For this review, use the dimensioned drawing (mm, ordinates from the lowest corner) and the shaded views. Coordinates: 2 decimals unless noted, no trailing zeros. Write each loop counter-clockwise with the first axis right and the second up, starting at its lowest first coordinate (ties: lowest second). Pieces come first, ordered by that corner, then holes. Notation, with made-up numbers: (-22.5, -39) - (23.5, -39) arc R15 ccw to (23.5, -28) - close; hole circle Ø1 at (50, 43). An arc over 180 degrees is marked (long way). One line per item, written item: value.
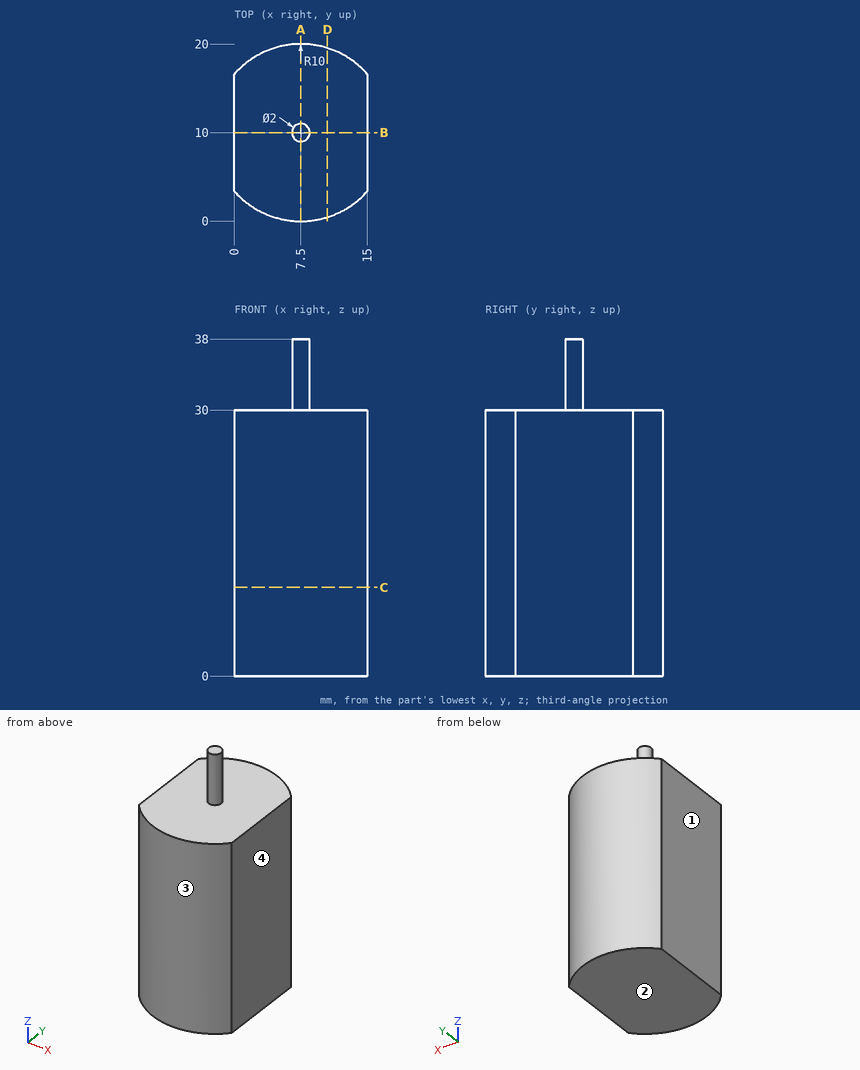
1. Insertion check: pin 1 Ø5 at (x, y) = (13.5, 13) entering from +Z; pin 2 Ø2 at (x, z) = (9, 30.5) entering from +Y. Each pin has a flat end and moves straight along its axis. Give the tip position at first contact, or say it passes through.
Answer block:
pin 1: stops at z = 30
pin 2: stops at y = 19.98
2. Consider section C-C, the plane z = 10. Write out the cut boundary in (x, y), then the cut area to 3 significant figures.
Answer block:
outline: (0, 3.39) arc R10 ccw to (15, 3.39) - (15, 16.61) arc R10 ccw to (0, 16.61) - close
area: 269 mm^2
3. Mouldability with a two-part tool opening along X and no side actions: class the marked faces 1, 2, 3 and 4 as released by +X, released by -X, zero draft, split by the parting line, or undercut.
Answer block:
face 1: released by -X
face 2: zero draft
face 3: split by the parting line
face 4: released by +X
4. Consider section D-D, the plane x = 10.5. Write out the cut boundary in (y, z).
Answer block:
outline: (0.46, 0) - (19.54, 0) - (19.54, 30) - (0.46, 30) - close
5. Consider section A-A, the plane x = 7.5. Write out the cut boundary in (y, z), then the cut area to 3 significant figures.
Answer block:
outline: (0, 0) - (20, 0) - (20, 30) - (11, 30) - (11, 38) - (9, 38) - (9, 30) - (0, 30) - close
area: 616 mm^2
6. Wall thickness on line 1 along Z through (x, y) = (11, 7); line 2 along Y through (x, z) = (7.5, 23.5); line 3 along X through (y, z) = (3, 2): over which ranges is each line inside the solid? List them lowest first.
Answer block:
line 1: z = 0 to 30
line 2: y = 0 to 20
line 3: x = 0.36 to 14.64
7. Consider section B-B, the plane y = 10. Write out the cut boundary in (x, z).
Answer block:
outline: (0, 0) - (15, 0) - (15, 30) - (8.5, 30) - (8.5, 38) - (6.5, 38) - (6.5, 30) - (0, 30) - close
